Can you work these out from the model? Positions are in its coordinate system, mm. Coordinates: 2 decimals unless noted, no trailing zeros. Order: outer loops, then holes, each group sorted by start corner. A loop starts at its lowest first (then second) coordinate and runs counter-clockwise, first axis right, second up. Notation, with made-up numbers: M 58,-5.75 L 94,-5.75 A23 cw 94,4.25 Z; hole C 79,75 d8. An arc over 180 degrees is marked long. Answer as a JSON object with one key per item and string values.
Autodesk Inventor part; units mm, degrees
ref_plane "YZ Plane" through (0, 0, 0) normal (1, 0, 0) x (0, 1, 0)
ref_plane "XZ Plane" through (0, 0, 0) normal (0, 1, 0) x (-1, 0, 0)
ref_plane "XY Plane" through (0, 0, 0) normal (0, 0, 1) x (1, 0, 0)
sketch "Sketch1" plane through (0, 0, 0) normal (0, 0, 1) x (1, 0, 0)
  line L0 (0, 0) -> (130, 0)
  line L1 (130, 0) -> (130, 130)
  line L2 (130, 130) -> (0, 130)
  line L3 (0, 130) -> (0, 0)
  line L4 (0, 130) -> (19.05, 130)
  line L5 (0, 130) -> (3.175, 130)
  dimension "d0" = 130
  dimension "d1" = 130
extrude "Extrusion1" add sketch "Sketch1" along normal blind 10
sketch "Sketch2" plane through (0, 0, 10) normal (0, 0, 1) x (1, 0, 0)
  line L0 (130, 130) -> (0, 130)
  line L1 (0, 130) -> (10, 130)
  line L2 (10, 130) -> (10, 10)
  line L3 (10, 10) -> (120, 10)
  line L4 (120, 10) -> (120, 120)
  line L5 (120, 120) -> (10, 120)
  circle A0 centre (10, 120) radius 5
  circle A1 centre (120, 120) radius 5
  circle A2 centre (120, 10) radius 5
  circle A3 centre (10, 10) radius 5
  point P0 (0, 0)
  dimension "d4" = 10
  dimension "d5" = 120
  dimension "d6" = 110
  dimension "d7" = 110
  dimension "d8" = 110
  dimension "d9" = 10
  dimension "d10" = 10
  dimension "d11" = 10
  dimension "d12" = 10
extrude "Extrusion2" cut sketch "Sketch2" against normal through all contours A0 L5 L2 | L2 A0 | L5 A0 L2 | A1 L4 L5 | L5 L4 A1 | A3 L3 L2 | L2 L3 A3 | A2 L3 L4 | L4 L3 A2
sketch "Sketch3" plane through (0, 0, 10) normal (0, 0, 1) x (1, 0, 0)
  line L0 (0, 0) -> (65, 0)
  line L1 (0, 0) -> (130, 0)
  line L2 (65, 0) -> (65, 30)
  circle A0 centre (65, 30) radius 5.5
  line L3 (130, 130) -> (0, 130)
  line L4 (0, 130) -> (65, 130)
  line L5 (65, 130) -> (65, 95)
  circle A1 centre (65, 95) radius 15
  dimension "d15" = 65
  dimension "d16" = 30
  dimension "d17" = 11
  dimension "d18" = 65
  dimension "d19" = 35
  dimension "d20" = 30
extrude "Extrusion3" cut sketch "Sketch3" against normal blind 10
properties part number "BOTTON"
Item 1: If we mould it in two halves opening along Y, with no side actions, what happens to faces 1 (the flat face through (66, 130, 5)), 2 (the flat face through (64, 66, 10)), 3 (the cylindrical face through (124.619, 118.085, 5.07))? For each: pulls with the +Y half, pulls with the -Y half, needs draft (parallel to the pull), parting line crosses it, or undercut.
Answers follow:
{"face 1": "pulls with the +Y half", "face 2": "needs draft", "face 3": "undercut"}
Item 2: I want a section at C-C, the plane z = 3.25. Write out the boundary of the cut face in (x, y), plus the area to 3 significant figures.
Answers follow:
{"outline": "M 0,0 L 130,0 L 130,130 L 0,130 Z; hole C 10,10 d10; hole C 10,120 d10; hole C 65,95 d30; hole C 65,30 d11; hole C 120,10 d10; hole C 120,120 d10", "area": "15,800 mm^2"}
Item 3: I want a section at B-B, the plane x = 120. Write out the boundary of the cut face in (y, z), plus the area to 3 significant figures.
Answers follow:
{"outline": "M 0,0 L 5,0 L 5,10 L 0,10 Z; M 15,0 L 115,0 L 115,10 L 15,10 Z; M 125,0 L 130,0 L 130,10 L 125,10 Z", "area": "1,100 mm^2"}
Item 4: I want a section at A-A, the plane y = 95. Write out the boundary of the cut face in (x, z), plus the area to 3 significant figures.
Answers follow:
{"outline": "M 0,0 L 50,0 L 50,10 L 0,10 Z; M 80,0 L 130,0 L 130,10 L 80,10 Z", "area": "1,000 mm^2"}
Item 5: I'm going to push a flat-ended pin straight in: pin 1 (8 mm diameter, centred on x = 120, y = 120, fed in from -Z). Where does the tip first touch, or does it pass through?
Answers follow:
{"pin 1": "passes through"}
Item 6: Please list where these lines run through material, in increasing order: line 1 (X direction, y = 10, z = 7); line 2 (X direction, y = 30, z = 6.25).
Answers follow:
{"line 1": "x = 0 to 5, 15 to 115, 125 to 130", "line 2": "x = 0 to 59.5, 70.5 to 130"}
